Could you check a few things on this drawing? It's one solid part, dimensions in mm from its lowest x, y, z. A direction names the side the tool comes from. Coordinates: 2 decimals unless noted, no trailing zeros. Write each loop counter-clockwise with the first axis right and the second up, starting at its lowest first coordinate (ties: lowest second). Pieces come first, ordered by that corner, then holes. Notation, with made-up numbers: M 67.25,-27.5 L 122.25,-27.5 A27 cw 122.25,1.5 Z; hole C -4.5,-4 d1. An arc over 180 degrees is marked long. Use a Markdown table: item, result.
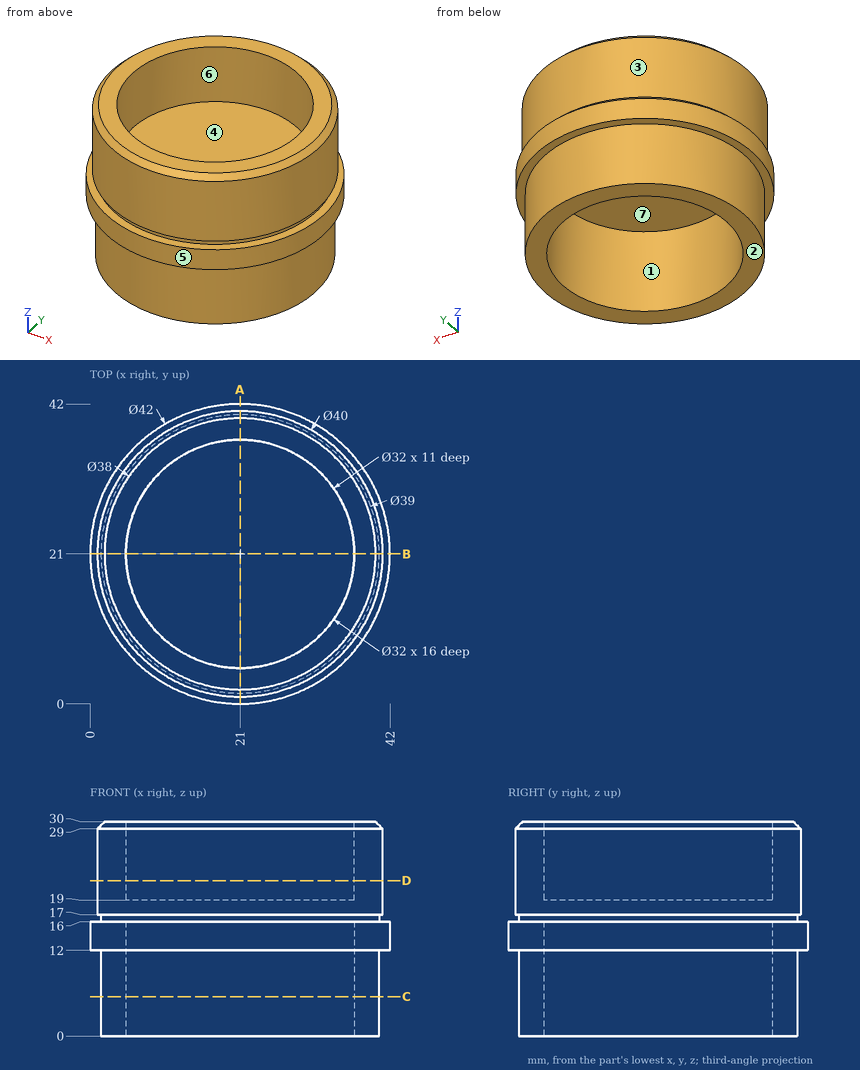
1. Which directions (+Z, -Z, +X, -X, +Y, -Y) give clear straight access to the entire face, cutting with the end or side of a thin tool? Please do the marked faces 5, 6 and 7.
Answers follow:
| item | result |
|---|---|
| face 5 | +Z, -Z |
| face 6 | +Z |
| face 7 | -Z |
2. I need wall thicknesses on probe 1 along Y at (x, z) = (21, 23.75); probe 2 along Y at (x, z) = (17.5, 24); probe 3 along Z at (x, y) = (13, 21). Which ranges of each line are inside material? Lowest first, please.
Answers follow:
| item | result |
|---|---|
| probe 1 | y = 1 to 5, 37 to 41 |
| probe 2 | y = 1.31 to 5.39, 36.61 to 40.69 |
| probe 3 | z = 16 to 19 |
3. Suppose I cut it at D-D on z = 21.75. Write out the boundary of the cut face in (x, y).
Answers follow:
| item | result |
|---|---|
| outline | C 21,21 d40; hole C 21,21 d32 |
4. Suppose I cut it at A-A on x = 21. Write out the boundary of the cut face in (y, z).
Answers follow:
| item | result |
|---|---|
| outline | M 0,12 L 1.5,12 L 1.5,0 L 5,0 L 5,16 L 37,16 L 37,0 L 40.5,0 L 40.5,12 L 42,12 L 42,16 L 40.5,16 L 40.5,17 L 41,17 L 41,29 L 40,30 L 37,30 L 37,19 L 5,19 L 5,30 L 2,30 L 1,29 L 1,17 L 1.5,17 L 1.5,16 L 0,16 Z |
5. Will these pins go through, and if not, where does the flat tip stop? pin 1 Ø1.5 at (x, z) = (30, 6) entering from +Y; pin 2 Ø1.5 at (x, z) = (9.5, 17) entering from -Y; pin 3 Ø12 at (x, z) = (35.5, 16.5) entering from -Y.
Answers follow:
| item | result |
|---|---|
| pin 1 | stops at y = 38.67 |
| pin 2 | stops at y = 4.13 |
| pin 3 | stops at y = 1.81 |
6. We'd pull the mould along Y, two halves only. Please class the marked faces 1, 2, 3 and 4: +Y half, -Y half, draft (parallel to the pull), parting line (faces both ways), or undercut.
Answers follow:
| item | result |
|---|---|
| face 1 | undercut |
| face 2 | draft |
| face 3 | parting line |
| face 4 | undercut |
7. Suppose I cut it at C-C on z = 5.5. Write out the boundary of the cut face in (x, y).
Answers follow:
| item | result |
|---|---|
| outline | C 21,21 d39; hole C 21,21 d32 |
